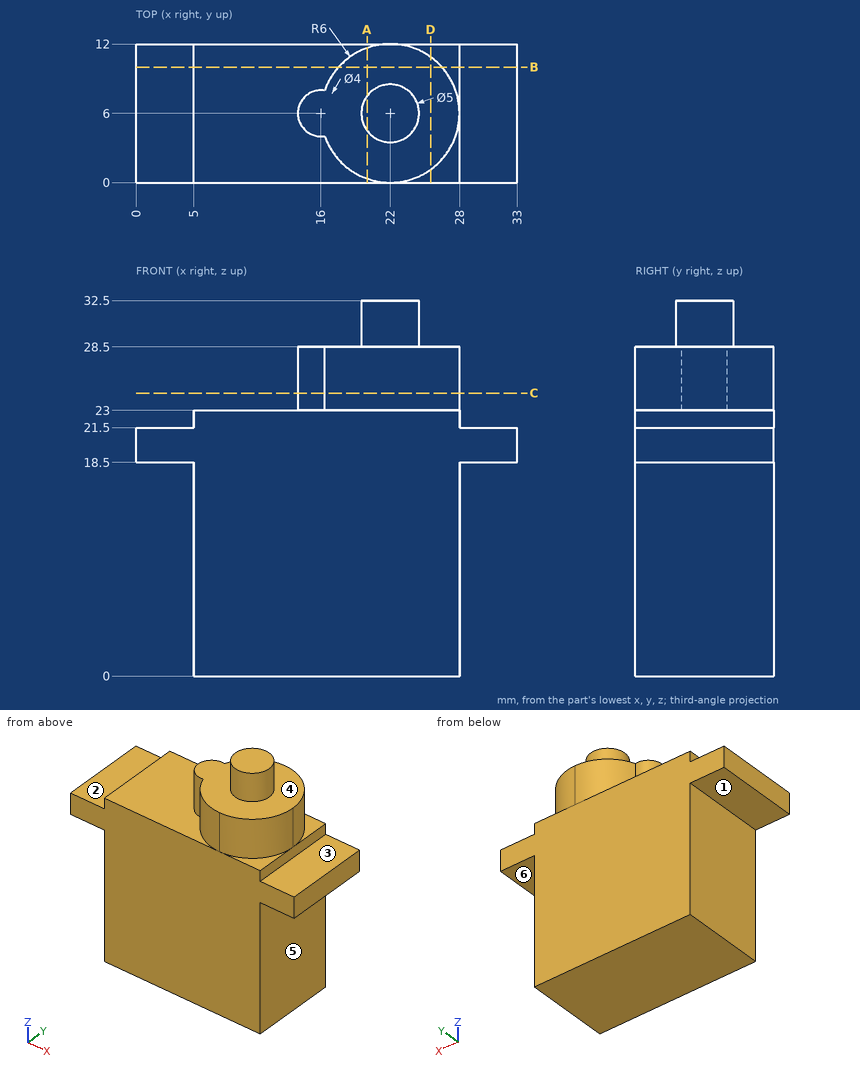
The figure shows three views and two pictorial views of one solid part (mm, origin at its lowest corner). Answer the questions. A direction names the side the tool comes from. Round coordinates to 2 decimals unless told otherwise and drop trailing zeros. Order: outer loops, then holes, each group sorted by start corner. A loop starts at its lowest first (then second) coordinate and runs counter-clockwise, first axis right, second up.
Q1. A cutting plane is placed at C-C, the plane z = 24.5. Determine the outline of the cut face in (x, y).
Solution:
outline: (16.33, 4.03) arc R6 ccw (long way) to (16.33, 7.97) arc R2 ccw (long way) to start
Q2. A cutting plane is placed at D-D, the plane x = 25.5. Determine the outline of the cut face in (y, z).
Solution:
outline: (0, 0) - (12, 0) - (12, 23) - (10.87, 23) - (10.87, 28.5) - (1.13, 28.5) - (1.13, 23) - (0, 23) - close
Q3. A cutting plane is placed at B-B, the plane y = 10. Determine the outline of the cut face in (x, z), then the cut area to 3 significant figures.
Solution:
outline: (0, 18.5) - (5, 18.5) - (5, 0) - (28, 0) - (28, 18.5) - (33, 18.5) - (33, 21.5) - (28, 21.5) - (28, 23) - (26.47, 23) - (26.47, 28.5) - (17.53, 28.5) - (17.53, 23) - (5, 23) - (5, 21.5) - (0, 21.5) - close
area: 608 mm2
Q4. A cutting plane is placed at A-A, the plane x = 20. Determine the outline of the cut face in (y, z).
Solution:
outline: (0, 0) - (12, 0) - (12, 23) - (11.66, 23) - (11.66, 28.5) - (7.5, 28.5) - (7.5, 32.5) - (4.5, 32.5) - (4.5, 28.5) - (0.34, 28.5) - (0.34, 23) - (0, 23) - close
Q5. The mould has two halves that part along Z. Classify the marked faces 4, 5 and 6: pulls with the +Z half, pulls with the -Z half, needs draft (parallel to the pull), parting line crosses it, or undercut.
Solution:
face 4: pulls with the +Z half
face 5: needs draft
face 6: pulls with the -Z half
Q6. A tool of negligible diameter and unlimited length cuts with its end or side. For the marked faces 1, 2 and 3, from which of +Z, -Z, +X, -X, +Y, -Y can it reach the whole face along a straight path? Write none if from no direction.
Solution:
face 1: -Z, -X, +Y, -Y
face 2: +Z, -X, +Y, -Y
face 3: +Z, +X, +Y, -Y
Q7. Find the intervals of material crossed by line 1 along X through (y, z) = (9.75, 13.5); line 2 along Z through (x, y) = (19.5, 6.5); line 3 along Z through (x, y) = (10, 3.25), in increasing order.
Solution:
line 1: x = 5 to 28
line 2: z = 0 to 28.5
line 3: z = 0 to 23
Q8. Given pin 1 Ø4 at (x, y) = (31, 9) entering from -Z; pin 2 Ø2 at (x, y) = (8, 6.5) entering from +Z; pin 3 Ø5 at (x, y) = (25.5, 4) entering from +Z; pin 4 Ø2.5 at (x, y) = (1.5, 4.5) entering from +Z, each flat-ended and moving along its own axis, determine where each tip first touches the part or whether it passes through.
Solution:
pin 1: stops at z = 18.5
pin 2: stops at z = 23
pin 3: stops at z = 32.5
pin 4: stops at z = 21.5
